from build123d import *

# Parameters (mm, degrees)
F0_W     = 257
F0_H     = 145
F0_W_2   = 205
F0_H_2   = 9
F1_DEPTH = 2.5
F2_W     = 20
F2_H     = 7.7
F3_DEPTH = 0.5


with BuildPart() as f1:
    # F0 (on Top) → F1 (new body)
    with BuildSketch(Plane.XY):
        Polygon((133, 76), (-135, 76), (-135, -81), (-91.5, -81), (113.5, -81), (133, -81), align=None)
        Rectangle(F0_W, F0_H, mode=Mode.SUBTRACT)
        Rectangle(F0_W, F0_H)
        with Locations((11, -85.5)):
            Rectangle(F0_W_2, F0_H_2)
    extrude(amount=F1_DEPTH)

    # F2 (on face) → F3 (cut)
    with BuildSketch(Plane.XY.offset(2.5)):
        with Locations((-36.5, -86.15)):
            Rectangle(F2_W, F2_H)
    extrude(amount=-F3_DEPTH, mode=Mode.SUBTRACT)


solid = f1.part
Design review of the part built by this model. Coordinates are the model's own, in mm. A direction names the side the tool comes from. Round coordinates to 2 decimals unless told otherwise and drop trailing zeros. Loops run counter-clockwise (first coordinate to the right, second up) from the corner with the lowest first, then second, coordinate; pieces in that order, holes last. Notation, with made-up numbers: (47.25, -3.75) -> (79.25, -3.75) arc R34 ccw to (79.25, 26.25) -> close; hole circle Ø5 at (72.5, 35.5). An arc over 180 degrees is marked (long way). Use one line per item in the form item = value. Start each with the question number.
Q1. Wall thickness on line 1 along Y through (x, z) = (-107, 0.3): over which ranges is the line inside the solid? List them lowest first. Write a range as [from, to].
Q2. Machinability: for faces 1 (the face through (-37, -86, 2)), 2 (the face through (-3, -6, 0)), which of the approach directions +Z, -Z, +X, -X, +Y, -Y give a long, thin tool a straight path to every point of the face, cutting with its end or side? Answer none if there is none.
Q3. We need section A-A on x = -96. Give the boundary of the cut face in (y, z), then the cut area to 4 significant figures.
Q4. For pin 1 Ø1.2 at (y, z) = (-87, 1) entering from +X; pin 2 Ø1.2 at (y, z) = (-84.5, 0.5) entering from -X; pin 3 Ø4 at (x, y) = (-32, -86.5) entering from +Z, all flat-tipped, find the tip position at first contact; note any pin that passes through.
Calculated:
q1.line_1 = [-81, 76]
q2.face_1 = +Z, -Y
q2.face_2 = -Z, +X, -X, +Y, -Y
q3.outline = (-81, 0) -> (76, 0) -> (76, 2.5) -> (-81, 2.5) -> close
q3.area = 392.5 mm²
q4.pin_1 = 113.5
q4.pin_2 = -91.5
q4.pin_3 = 2
